```python
from build123d import *

# Parameters (mm, degrees)
EXTRUDE_1_DEPTH     = 2
SKETCH_2_W          = 20.3
SKETCH_2_H          = 3
EXTRUDE_2_DEPTH     = 15
SKETCH_3_R          = 1.5
CUT_EXTRUDE_1_DEPTH = 15
SKETCH_6_R          = 1.25
CUT_EXTRUDE_3_DEPTH = 10
EXTRUDE_3_DEPTH     = 2


with BuildPart() as part:
    # 草图1 → 凸台-拉伸1 (new body)
    with BuildSketch(Plane(origin=(0, 0, 0), x_dir=(1, 0, 0), z_dir=(0, 1, 0))):
        Polygon((8, 47.06), (0, 47.06), (0, 44.06), (0, 0), (20.3, 0), (20.3, 35.06), (8, 35.06), align=None)
        with BuildLine():
            ThreePointArc((4, 44.06), (3, 43.06), (2, 44.06))
            ThreePointArc((2, 44.06), (3, 45.06), (4, 44.06))
        make_face(mode=Mode.SUBTRACT)
    extrude(amount=EXTRUDE_1_DEPTH)

    # 草图2 → 凸台-拉伸2 (add)
    with BuildSketch(Plane(origin=(0, 2, 0), x_dir=(1, 0, 0), z_dir=(0, 1, 0))):
        with Locations((10.15, 1.5)):
            Rectangle(SKETCH_2_W, SKETCH_2_H)
    extrude(amount=EXTRUDE_2_DEPTH)

    # 草图3 → 切除-拉伸1 (cut)
    with BuildSketch(Plane(origin=(0, 0, -3), x_dir=(-1, 0, 0), z_dir=(0, 0, -1))):
        with Locations((-15.3, 13.75)):
            Circle(SKETCH_3_R)
        with Locations((-15.3, 5.25)):
            Circle(SKETCH_3_R)
        with Locations((-5, 13.75)):
            Circle(SKETCH_3_R)
        with Locations((-5, 5.25)):
            Circle(SKETCH_3_R)
    extrude(amount=-CUT_EXTRUDE_1_DEPTH, mode=Mode.SUBTRACT)

    # 草图6 → 切除-拉伸3 (cut)
    with BuildSketch(Plane.XZ):
        with Locations(Location((17.3, -6, 0), (0, 0, 270))):
            Circle(SKETCH_6_R)
    extrude(amount=-CUT_EXTRUDE_3_DEPTH, mode=Mode.SUBTRACT)

    # 草图7 → 凸台-拉伸3 (add, symmetric)
    with BuildSketch(Plane.ZY.offset(-10.15)):
        Polygon((-3, 17), (-3, 2), (-32.000508887, 2), align=None)
    extrude(amount=EXTRUDE_3_DEPTH, both=True)


solid = part.part
```
Geometry check sheet. Reference: the model listing, model coordinates, mm. A direction names the side the tool comes from. Give positions to 0.01 mm unless a question says otherwise; leave off trailing zeros. Write each loop counter-clockwise with the first axis right and the second up, starting at its lowest first coordinate (ties: lowest second). Pieces come first, ordered by that corner, then holes. Notation, with made-up numbers: (65, -33) - (103, -33) arc R33 cw to (103, -2) - close; hole circle Ø11 at (64, 5.25). An arc over 180 degrees is marked (long way). Use a Markdown table: item, result.
Q1. Section check A-A, the plane x = 15.3. Enter the section's corners in (y, z).
Computed:
| item | result |
|---|---|
| outline | (0, -35.06) - (2, -35.06) - (2, -3) - (3.75, -3) - (3.75, 0) - (0, 0) - close; (6.75, -3) - (12.25, -3) - (12.25, 0) - (6.75, 0) - close; (15.25, -3) - (17, -3) - (17, 0) - (15.25, 0) - close |
Q2. Section check B-B, the plane z = -44.06. Enter the section's corners in (x, y), then the cut area to 3 significant figures.
Computed:
| item | result |
|---|---|
| outline | (0, 0) - (2, 0) - (2, 2) - (0, 2) - close; (4, 0) - (8, 0) - (8, 2) - (4, 2) - close |
| area | 12.0 mm² |
Q3. Section check C-C, the plane y = 1.5. Enter the section's corners in (x, z), then the cut area to 3 significant figures.
Computed:
| item | result |
|---|---|
| outline | (0, -47.06) - (8, -47.06) - (8, -35.06) - (20.3, -35.06) - (20.3, 0) - (0, 0) - close; hole circle Ø2 at (3, -44.06); hole circle Ø2.5 at (17.3, -6) |
| area | 800 mm² |
Q4. Set-up check for faces 1 (the face through (4, 9, -3)), 2 (the face through (16.8, 5.3, -1.5)), 3 (the face through (3.13, 0.99, -45.05)), 4 (the face through (16, 9, -3)), 5 (the face through (8, 2, -20)): record each of +Z, -Z, +X, -X, +Y, -Y from which the full face is reachable in a straight line by a thin tool's end or side.
Computed:
| item | result |
|---|---|
| face 1 | -Z, -X, +Y |
| face 2 | +Z, -Z |
| face 3 | +Y, -Y |
| face 4 | -Z, +X, +Y |
| face 5 | -Z, +Y |
Q5. Thickness scan on L1, parallel to Y at x = 5, z = -1.85; L2, parallel to X at y = 1.05, z = -44.06; L3, parallel to Z at x = 3, y = 0.4. Record the ranges inside material, lowest first. Write a range as [from, to].
Computed:
| item | result |
|---|---|
| L1 | y = [0, 3.75], [6.75, 12.25], [15.25, 17] |
| L2 | x = [0, 2], [4, 8] |
| L3 | z = [-47.06, -45.06], [-43.06, 0] |
Q6. Go/stop test with flat-tipped pins: P1, Ø4.5, axis at y = 9, z = -22.5, coming from the +X side; P2, Ø1, axis at x = 15, y = 10.5, coming from the -Z side; P3, Ø2, axis at x = 12.5, y = 0.5, coming from the -Z side. Record where each tip stops, or that it passes through.
Computed:
| item | result |
|---|---|
| P1 | stops at x = 12.15 |
| P2 | stops at z = -3 |
| P3 | stops at z = -35.06 |
Q7. Section check D-D, the plane x = 3. Enter the section's corners in (y, z).
Computed:
| item | result |
|---|---|
| outline | (0, -47.06) - (2, -47.06) - (2, -45.06) - (0, -45.06) - close; (0, -43.06) - (2, -43.06) - (2, -3) - (17, -3) - (17, 0) - (0, 0) - close |
Q8. Draft check along Z on faces 6 (the face through (16.08, 0.99, -5.73)), 7 (the face through (8.15, 6, -11)), 8 (the face through (14, 1, -35.06)). Enter one of: pulls with the +Z half, pulls with the -Z half, needs draft (parallel to the pull), parting line crosses it, or undercut.
Computed:
| item | result |
|---|---|
| face 6 | undercut |
| face 7 | needs draft |
| face 8 | pulls with the -Z half |
